```python
from build123d import *

# Parameters (mm, degrees)
SKETCH1_R           = 3
SKETCH1_R_2         = 0.75
SKETCH1_R_3         = 0.5
SKETCH1_W           = 7.75
SKETCH1_H           = 4
BOSS_EXTRUDE1_DEPTH = 4


with BuildPart() as part:
    # Sketch1 → Boss-Extrude1 (new body)
    with BuildSketch(Plane.XY):
        Polygon((8.000003067, 19.999998036), (31.500003067, 19.999998036), (39.500003067, 11.999998036), (39.500003067, 7.999998036), (31.500003067, -1.964e-06), (8.000003067, -1.964e-06), (3.067e-06, 7.999998036), (3.067e-06, 11.999998036), align=None)
        with Locations((19.750003067, 9.999998036)):
            Circle(SKETCH1_R, mode=Mode.SUBTRACT)
        with Locations((18.000003067, 16.999998036)):
            Circle(SKETCH1_R_2, mode=Mode.SUBTRACT)
        with Locations((21.500003067, 16.999998036)):
            Circle(SKETCH1_R_2, mode=Mode.SUBTRACT)
        with Locations((18.000003067, 3.499998036)):
            Circle(SKETCH1_R_3, mode=Mode.SUBTRACT)
        with Locations((21.500003067, 3.499998036)):
            Circle(SKETCH1_R_3, mode=Mode.SUBTRACT)
        with Locations((9.875003067, 9.999998036)):
            Rectangle(SKETCH1_W, SKETCH1_H, mode=Mode.SUBTRACT)
        with Locations((29.625003067, 9.999998036)):
            Rectangle(SKETCH1_W, SKETCH1_H, mode=Mode.SUBTRACT)
    extrude(amount=BOSS_EXTRUDE1_DEPTH)


solid = part.part
```
Design review of the part built by this model. Coordinates are the model's own, in mm. A direction names the side the tool comes from. Coordinates: 2 decimals unless noted, no trailing zeros. Order: outer loops, then holes, each group sorted by start corner. A loop starts at its lowest first (then second) coordinate and runs counter-clockwise, first axis right, second up. Notation, with made-up numbers: (44, -16.5) -> (93, -16.5) arc R29 ccw to (93, 18.5) -> close; hole circle Ø7 at (-0.75, 12). An arc over 180 degrees is marked (long way). One line per item, written item: value. Start each with the question number.
Q1. Tool access review of faces 5 (the flat face through (35.6, 4.1, 2)), 6 (the flat face through (30, 8, 2)): name each direction out of +Z, -Z, +X, -X, +Y, -Y from which nothing blocks a thin tool from reaching the whole face with its end or side.
Q2. For probe 1 along Y at (x, z) = (27, 3.15); probe 2 along Y at (x, z) = (21.5, 1.3); probe 3 along Y at (x, z) = (22.5, 3.3), list the stretches that pass through material, from the lowest coordinate up.
Q3. Take a section at D-D, the plane y = 14. State the section outline as (x, z) points.
Q4. Take a section at C-C, the plane y = 7.5. State the section outline as (x, z) points.
Q5. Take a section at B-B, the plane z = 0.7. State the section outline as (x, y) points, then the cut area to 3 significant figures.
Q6. Mouldability with a two-part tool opening along X and no side actions: class faces 1 (the flat face through (4, 16, 2)), 2 (the flat face through (35.4, 16.1, 2)), 3 (the flat face through (16, 10, 0)), 4 (the flat face through (10, 12, 2)) as pulls with the +X half, pulls with the -X half, needs draft (parallel to the pull), parting line crosses it, or undercut.
Q7. Take a section at A-A, the plane x = 33. State the section outline as (y, z) points, then the cut area to 3 significant figures.
Q8. Insertion check: pin 1 Ø1.5 at (y, z) = (18, 2.5) entering from -X. The pin has a flat end and moves straight along its axis. Give the tip position at first contact, or say it passes through.
Values follow:
1. face 5: +Z, -Z, +X, -Y
1. face 6: +Z, -Z
2. probe 1: y = 0 to 8, 12 to 20
2. probe 2: y = 0 to 3, 4 to 7.56, 12.44 to 16.25, 17.75 to 20
2. probe 3: y = 0 to 8.8, 11.2 to 20
3. outline: (2, 0) -> (37.5, 0) -> (37.5, 4) -> (2, 4) -> close
4. outline: (0.5, 0) -> (18.09, 0) -> (18.09, 4) -> (0.5, 4) -> close; (21.41, 0) -> (39, 0) -> (39, 4) -> (21.41, 4) -> close
5. outline: (0, 8) -> (8, 0) -> (31.5, 0) -> (39.5, 8) -> (39.5, 12) -> (31.5, 20) -> (8, 20) -> (0, 12) -> close; hole (6, 8) -> (13.75, 8) -> (13.75, 12) -> (6, 12) -> close; hole circle Ø6 at (19.75, 10); hole circle Ø1.5 at (18, 17); hole circle Ø1 at (18, 3.5); hole circle Ø1.5 at (21.5, 17); hole circle Ø1 at (21.5, 3.5); hole (25.75, 8) -> (33.5, 8) -> (33.5, 12) -> (25.75, 12) -> close
5. area: 567 mm2
6. face 1: pulls with the -X half
6. face 2: pulls with the +X half
6. face 3: needs draft
6. face 4: undercut
7. outline: (1.5, 0) -> (8, 0) -> (8, 4) -> (1.5, 4) -> close; (12, 0) -> (18.5, 0) -> (18.5, 4) -> (12, 4) -> close
7. area: 52.0 mm2
8. pin 1: stops at x = 5.25
